Here's the drawing with two shaded views (mm, measured from the low corner). I have some questions. A direction names the side the tool comes from. Coordinates: 2 decimals unless noted, no trailing zeros. Loops run counter-clockwise (first coordinate to the right, second up) from the corner with the lowest first, then second, coordinate; pieces in that order, holes last. Notation, with made-up numbers: (-7.75, 40) -> (43.25, 40) arc R19 cw to (43.25, 48) -> close; hole circle Ø10 at (2, 13.5). An arc over 180 degrees is marked (long way). Answer as a JSON object with one key per item and string values. Group by question number.
1) If we mould it in two halves opening along Y, with no side actions, what happens to the marked faces 4, 5 and 6? For each: +Y half, -Y half, draft (parallel to the pull), parting line (faces both ways), or undercut.
2) I want a section at C-C (z = 19). Write out the boundary of the cut face in (x, y), then the cut area to 3 significant figures.
3) I'm going to push flat-ended pins straight in: pin 1 (5.5 mm diameter, centred on x = 37.56, y = 37.56, fed in from +Z); pin 2 (3 mm diameter, centred on y = 8.5, z = 7.5, fed in from -X); pin 3 (4 mm diameter, centred on y = 26.5, z = 4, fed in from -X); pin 4 (2.5 mm diameter, centred on x = 6.44, y = 37.56, fed in from +Z). Where does each tip first touch, or does it pass through?
4) Which directions (+Z, -Z, +X, -X, +Y, -Y) give clear straight access to the entire face, cutting with the end or side of a thin tool? Please do the marked faces 1, 2 and 3.
5) I want a section at A-A (x = 22). Write out the boundary of the cut face in (y, z), then the cut area to 3 significant figures.
6) I need wall thicknesses on probe 1 along Y at (x, z) = (37.5, 26.25); probe 2 along X at (y, z) = (8.5, 25.75) (1 decimal); probe 3 along Z at (x, y) = (3, 17). Which ranges of each line are inside material? Lowest first, please. Write a range as [from, to].
7) I want a section at D-D (y = 36.5). Count the separate pieces of the cut face and the enclosed holes in it.
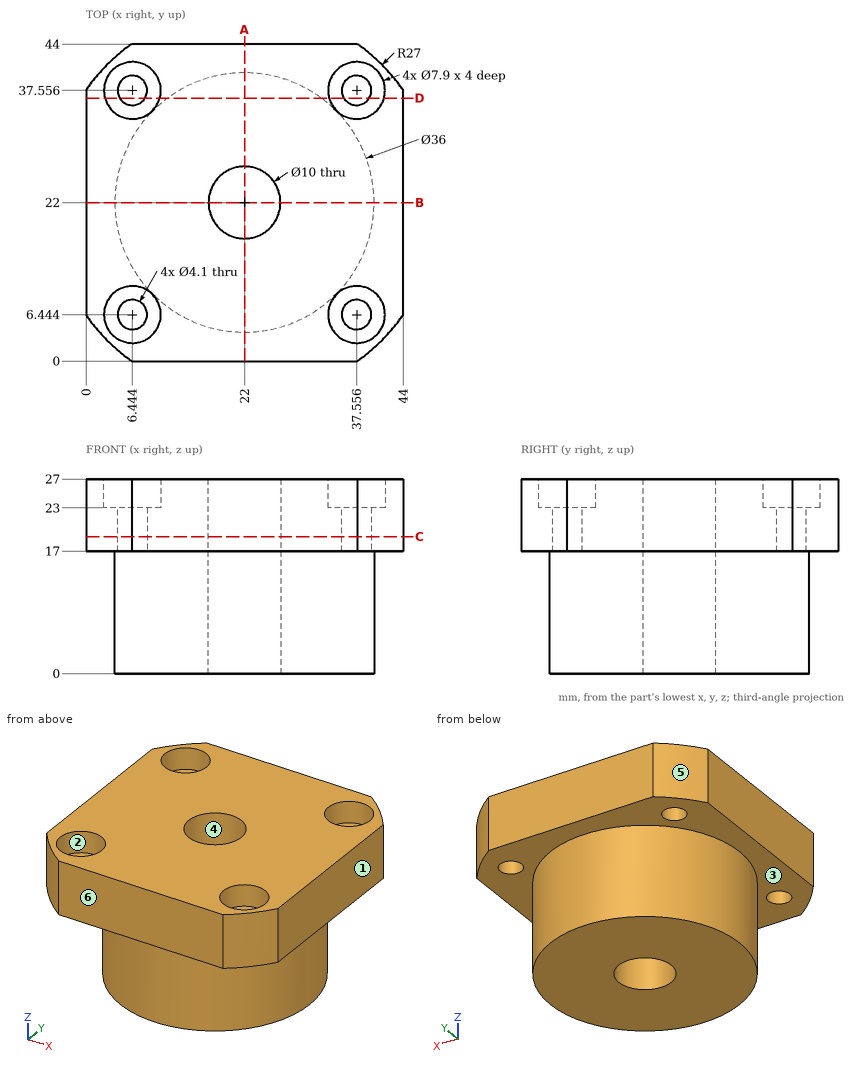
Determined:
{
 "1": {"face 4": "undercut", "face 5": "+Y half", "face 6": "-Y half"},
 "2": {"outline": "(0, 6.35) arc R27 ccw to (6.35, 0) -> (37.65, 0) arc R27 ccw to (44, 6.35) -> (44, 37.65) arc R27 ccw to (37.65, 44) -> (6.35, 44) arc R27 ccw to (0, 37.65) -> close; hole circle Ø4.1 at (6.44, 6.44); hole circle Ø4.1 at (6.44, 37.56); hole circle Ø10 at (22, 22); hole circle Ø4.1 at (37.56, 6.44); hole circle Ø4.1 at (37.56, 37.56)", "area": "1,730 mm^2"},
 "3": {"pin 1": "z = 23", "pin 2": "x = 8.58", "pin 3": "x = 4.17", "pin 4": "through"},
 "4": {"face 1": "+Z, -Z, +X, +Y, -Y", "face 2": "+Z", "face 3": "-Z"},
 "5": {"outline": "(0, 17) -> (4, 17) -> (4, 0) -> (17, 0) -> (17, 27) -> (0, 27) -> close; (27, 0) -> (40, 0) -> (40, 17) -> (44, 17) -> (44, 27) -> (27, 27) -> close", "area": "782 mm^2"},
 "6": {"probe 1": "[0, 2.49], [10.39, 33.61], [41.51, 44]", "probe 2": "[0, 3.1], [9.8, 34.2], [40.9, 44]", "probe 3": "[17, 27]"},
 "7": {"separate pieces": "3", "enclosed holes": "0"}
}
